The model under review builds one solid part; all positions refer to its coordinate system, in mm. Face numbers are marked on the shaded views. A direction names the side the tool comes from. Coordinates: 2 decimals unless noted, no trailing zeros. Write each loop counter-clockwise with the first axis right and the second up, starting at its lowest first coordinate (ties: lowest second). Pieces come first, ordered by that corner, then holes.
1) Add section B-B, the plane y = 4.75. State the section outline as (x, z) points, then the cut area to 3 significant figures.
2) For line 1 (X direction, y = 0, z = 0.9); line 2 (Y direction, x = -1.25, z = 1.4); line 3 (Y direction, x = -3, z = 1.25), list the stretches that pass through material, from the lowest coordinate up.
3) Machinability: for the marked faces 1 and 2, which of the approach directions +Z, -Z, +X, -X, +Y, -Y give a long, thin tool a straight path to every point of the face, cutting with its end or side? Answer none if there is none.
4) Add section D-D, the plane y = -4.25. State the section outline as (x, z) points, then the cut area to 3 significant figures.
5) Add section C-C, the plane z = 1.35. State the section outline as (x, y) points.
6) Add section A-A, the plane x = 2.75. State the section outline as (y, z) points.
7) For P1, Ø1, axis at y = 4, z = 1, coming from the +X side; P2, Ø5, axis at x = 0, y = 0, coming from the -Z side, all flat-tipped, find the tip position at first contact; note any pin that passes through.
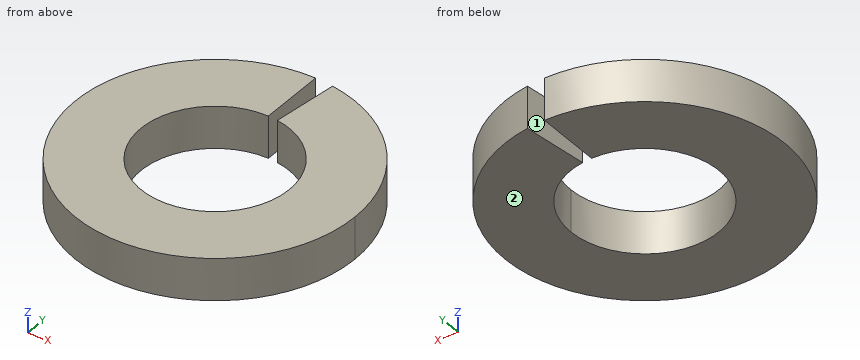
from build123d import *

# Parameters (mm, degrees)
SKETCH1_R      = 6.1595
SKETCH1_R_2    = 3.2639
EXTRUDE1_DEPTH = 1.8542
EXTRUDE2_DEPTH = 1.8542


with BuildPart() as part:
    # Sketch1 → Extrude1 (new body)
    with BuildSketch(Plane.XY):
        Circle(SKETCH1_R)
        Circle(SKETCH1_R_2, mode=Mode.SUBTRACT)
    extrude(amount=EXTRUDE1_DEPTH)

    # Sketch2 → Extrude2 (cut)
    with BuildSketch(Plane.XY.offset(1.8542)):
        with BuildLine():
            Line((0, 0), (0, 6.1595))
            ThreePointArc((0, 6.1595), (0.393778969, 6.146899899), (0.785946881, 6.109151148))
            Line((0.785946881, 6.109151148), (0, 0))
        make_face()
    extrude(amount=-EXTRUDE2_DEPTH, mode=Mode.SUBTRACT)


solid = part.part
Geometry results:
1. outline: (-3.92, 0) - (0, 0) - (0, 1.85) - (-3.92, 1.85) - close; (0.61, 0) - (3.92, 0) - (3.92, 1.85) - (0.61, 1.85) - close
1. area: 13.4 mm2
2. line 1: x = -6.16 to -3.26, 3.26 to 6.16
2. line 2: y = -6.03 to -3.02, 3.02 to 6.03
2. line 3: y = -5.38 to -1.29, 1.29 to 5.38
3. face 1: +Z, -Z, +Y
3. face 2: -Z, +X, -X, +Y, -Y
4. outline: (-4.46, 0) - (4.46, 0) - (4.46, 1.85) - (-4.46, 1.85) - close
4. area: 16.5 mm2
5. outline: (0, 3.26) - (0, 6.16) arc R6.16 ccw (long way) to (0.79, 6.11) - (0.42, 3.24) arc R3.26 cw (long way) to start
6. outline: (-5.51, 0) - (-1.76, 0) - (-1.76, 1.85) - (-5.51, 1.85) - close; (1.76, 0) - (5.51, 0) - (5.51, 1.85) - (1.76, 1.85) - close
7. P1: stops at x = 5.07
7. P2: passes through
